Design review of the part built by this model. Coordinates are the model's own, in mm. Face numbers are marked on the shaded views. A direction names the side the tool comes from. Round coordinates to 2 decimals unless told otherwise and drop trailing zeros. Write each loop counter-clockwise with the first axis right and the second up, starting at its lowest first coordinate (ties: lowest second). Pieces come first, ordered by that corner, then holes. Notation, with made-up numbers: M 45,85.25 L 53,85.25 A21 ccw 53,101.25 Z; hole C 5.5,60 d8. An arc over 180 degrees is marked long. Use CSV: the item, a comma, the result in double quotes.
from build123d import *

# Parameters (mm, degrees)
ESBO_O1_W                = 30
ESBO_O1_H                = 30
RESSALTO_EXTRUS_O1_DEPTH = 22.775
CORTE_EXTRUS_O1_DEPTH    = 31
ESBO_O3_OUTSIDE_W        = 48.998
ESBO_O3_OUTSIDE_H        = 41.63
ESBO_O3_OUTSIDE_W_2      = 30
ESBO_O3_OUTSIDE_H_2      = 30
CORTE_EXTRUS_O2_DEPTH    = 20.723728571
RESSALTO_EXTRUS_O2_DEPTH = 30
ESBO_O5_R                = 3.95
CORTE_EXTRUS_O3_DEPTH    = 25.958558799
CORTE_EXTRUS_O5_START    = -8
ESBO_O8_R                = 6
CORTE_EXTRUS_O5_DEPTH    = 25
RESSALTO_EXTRUS_O6_DEPTH = 30
CORTE_EXTRUS_O11_DEPTH   = 26
ESBO_O19_R               = 6.35
CORTE_EXTRUS_O12_DEPTH   = 3.5
ESBO_O20_R               = 3
CORTE_EXTRUS_O13_DEPTH   = 26


with BuildPart() as part:
    # Esboço1 → Ressalto-extrusão1 (new body)
    with BuildSketch(Plane(origin=(0, 0, 0), x_dir=(1, 0, 0), z_dir=(0, 1, 0))):
        Rectangle(ESBO_O1_W, ESBO_O1_H)
    extrude(amount=RESSALTO_EXTRUS_O1_DEPTH)

    # Esboço2 → Corte-extrusão1 (cut, through all)
    with BuildSketch(Plane.XY.offset(15)):
        Polygon((-15, 0), (15, 17.320508076), (15, 0), align=None)
    extrude(amount=-CORTE_EXTRUS_O1_DEPTH, mode=Mode.SUBTRACT)

    # Esboço3 outside → Corte-extrusão2 (cut, through all)
    with BuildSketch(Plane(origin=(-3.75, 6.495190528, 0), x_dir=(0.866025404, 0.5, 0), z_dir=(0.5, -0.866025404, 0))):
        with Locations((5.694, 0)):
            Rectangle(ESBO_O3_OUTSIDE_W, ESBO_O3_OUTSIDE_H)
        with Locations((4.330127019, 0)):
            Rectangle(ESBO_O3_OUTSIDE_W_2, ESBO_O3_OUTSIDE_H_2, mode=Mode.SUBTRACT)
    extrude(amount=-CORTE_EXTRUS_O2_DEPTH, mode=Mode.SUBTRACT)

    # Esboço4 → Ressalto-extrusão2 (add)
    with BuildSketch(Plane.XY.offset(15)):
        Polygon((-25.469660456, 22.775), (-15, 4.641016151), (-15, 22.775), align=None)
    extrude(amount=-RESSALTO_EXTRUS_O2_DEPTH)

    # Esboço5 → Corte-extrusão3 (cut, through all)
    with BuildSketch(Plane(origin=(-3.75, 6.495190528, 0), x_dir=(-0.866025404, -0.5, 0), z_dir=(0.5, -0.866025404, 0))):
        with Locations((-4.330131096, -4.077e-06)):
            Circle(ESBO_O5_R)
    extrude(amount=-CORTE_EXTRUS_O3_DEPTH, mode=Mode.SUBTRACT)

    # Esboço8 → Corte-extrusão5 (cut)
    with BuildSketch(Plane(origin=(-3.75, 6.495190528, 0), x_dir=(0.866025404, 0.5, 0), z_dir=(0.5, -0.866025404, 0)).offset(CORTE_EXTRUS_O5_START)):
        with Locations((4.330131096, 4.077e-06)):
            Circle(ESBO_O8_R)
    extrude(amount=-CORTE_EXTRUS_O5_DEPTH, mode=Mode.SUBTRACT)

    # Esboço16 → Ressalto-extrusão6 (add)
    with BuildSketch(Plane.XY.offset(15)):
        Polygon((9.171355695, 22.775), (30.157076086, 22.775), (30.157076086, 15.275), (11.457076086, 15.275), align=None)
    extrude(amount=-RESSALTO_EXTRUS_O6_DEPTH)

    # Esboço17 → Corte-extrusão11 (cut)
    with BuildSketch(Plane(origin=(0, 22.775, 0), x_dir=(1, 0, 0), z_dir=(0, 1, 0))):
        with BuildLine():
            Line((5.221968449, -14.998459918), (5.221968449, -42.526473986))
            Line((5.221968449, -42.526473986), (-49.914065742, -42.526473986))
            Line((-49.914065742, -42.526473986), (-49.914065742, 15))
            Line((-49.914065742, 15), (-24.474999573, 15))
            ThreePointArc((-24.474999573, 15), (-15.795068431, -6.105787356), (5.221968449, -14.998459918))
        make_face()
    extrude(amount=-CORTE_EXTRUS_O11_DEPTH, mode=Mode.SUBTRACT)

    # Esboço19 → Corte-extrusão12 (cut)
    with BuildSketch(Plane.XZ.offset(-15.275)):
        with Locations((20.807076086, 0)):
            Circle(ESBO_O19_R)
    extrude(amount=-CORTE_EXTRUS_O12_DEPTH, mode=Mode.SUBTRACT)

    # Esboço20 → Corte-extrusão13 (cut)
    with BuildSketch(Plane.XZ.offset(-18.775)):
        with Locations((20.807076086, 0)):
            Circle(ESBO_O20_R)
    extrude(amount=-CORTE_EXTRUS_O13_DEPTH, mode=Mode.SUBTRACT)


solid = part.part
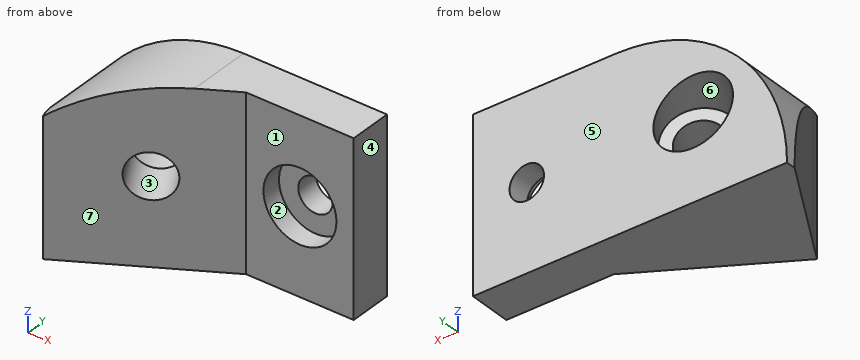
1) For pin 1 Ø6.5 at (x, z) = (21, 1.5) entering from -Y (3 decimals); pin 2 Ø1 at (y, z) = (9, -1.5) entering from +X; pin 3 Ø7 at (x, z) = (20.81, 0) entering from +Y (3 decimals); pin 4 Ø10 at (y, z) = (4.5, 1.5) entering from -X, all flat-tipped, find the tip position at first contact; note any pin that passes through.
Answers:
pin 1,"y = 18.775"
pin 2,"x = -4.02"
pin 3,"y = 22.775"
pin 4,"x = -17.81"
2) Wall thickness on line 1 along X through (y, z) = (21, 2.5); line 2 along X through (y, z) = (18, -2); line 3 along Z through (x, y) = (25.5, 17.5): over which ranges is each line inside the solid? List them lowest first. Write a range as [from, to].
Answers:
line 1,"[-18.84, -13.42], [-0.83, 19.15], [22.47, 30.16]"
line 2,"[-21.51, -11.92], [0.18, 14.78], [26.83, 30.16]"
line 3,"[-15, -4.28], [4.28, 15]"
3) The part is to be moulded in two halves that separate along Y. For the marked faces 4, 5, 6 and 7, say which applies: released by +Y, released by -Y, zero draft, split by the parting line, or undercut.
Answers:
face 4,"zero draft"
face 5,"released by +Y"
face 6,"undercut"
face 7,"released by -Y"
4) Add section B-B on z = -9. Write out the cut boundary in (x, y) (3 decimals).
Answers:
outline,"M -23.869,20.002 L -12.99,1.16 L 11.457,15.275 L 30.157,15.275 L 30.157,22.775 L -23.869,22.775 Z"
5) Machinability: for the marked faces 1, 2 and 3, which of the approach directions +Z, -Z, +X, -X, +Y, -Y give a long, thin tool a straight path to every point of the face, cutting with its end or side? Answer none if there is none.
Answers:
face 1,"+Z, -Z, +X, -Y"
face 2,"-Y"
face 3,"none"
6) Add section A-A on x = 22. Write out the cut boundary in (y, z) (3 decimals).
Answers:
outline,"M 15.275,-15 L 22.775,-15 L 22.775,-2.753 L 18.775,-2.753 L 18.775,-6.237 L 15.275,-6.237 Z; M 15.275,6.237 L 18.775,6.237 L 18.775,2.753 L 22.775,2.753 L 22.775,15 L 15.275,15 Z"
7) Add section C-C on y = 20. Give the number of separate pieces and of enclosed holes in the cut face, then the cut area to 3 significant figures.
Answers:
separate pieces,"1"
enclosed holes,"2"
area,"1,280 mm²"
8) Add section D-D on x = 9.5. Write out the cut boundary in (y, z) (3 decimals).
Answers:
outline,"M 14.145,-15 L 22.775,-15 L 22.775,15 L 14.145,15 Z"
